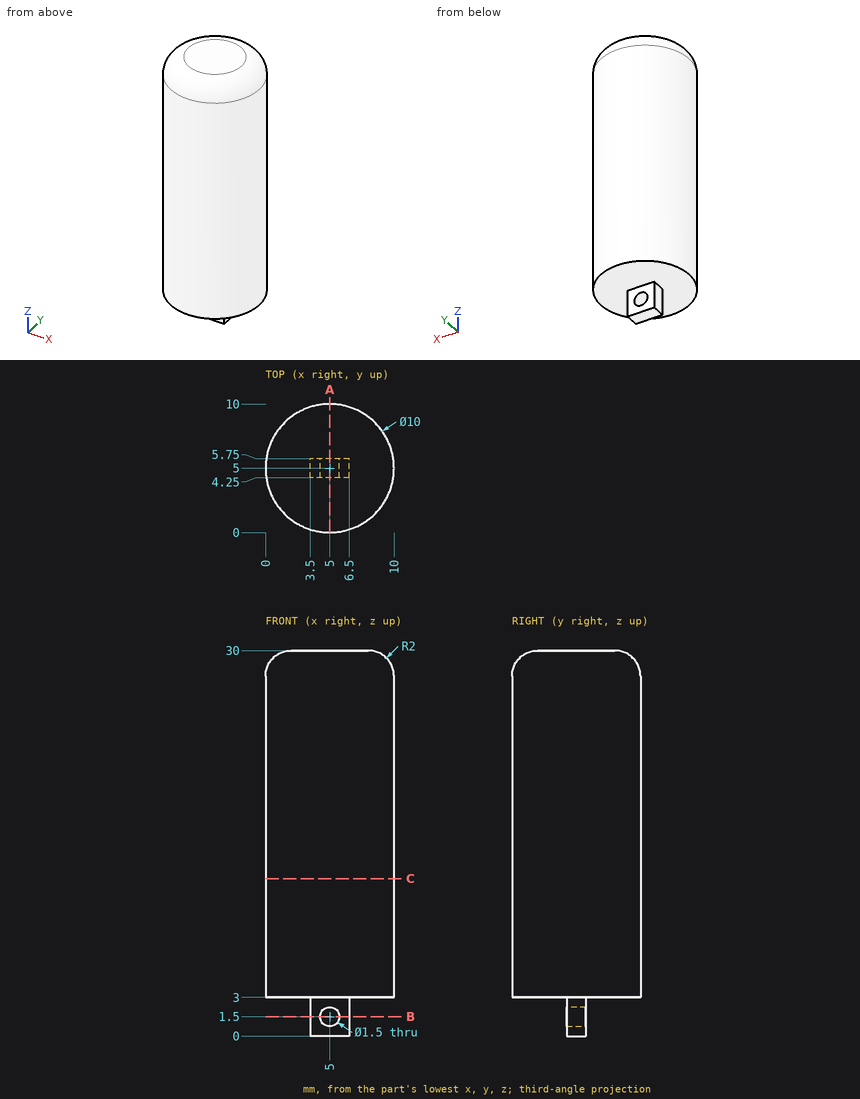
Print and shaded views of the part. All mm, measured from the part's lowest x, y and z. Round coordinates to 2 decimals unless told otherwise and drop trailing zeros. Write each loop counter-clockwise with the first axis right and the second up, starting at its lowest first coordinate (ties: lowest second). Pieces come first, ordered by that corner, then holes. Notation, with made-up numbers: (20.5, 86) - (77.5, 86) arc R34 cw to (77.5, 116) - close; hole circle Ø8 at (40, 5). An arc over 180 degrees is marked (long way). One line per question, with ' | ' between items.
1. Band-saw the part on B-B, the plane z = 1.5. Write the cut outline in (x, y).
Results are:
outline: (3.5, 4.25) - (4.25, 4.25) - (4.25, 5.75) - (3.5, 5.75) - close; (5.75, 4.25) - (6.5, 4.25) - (6.5, 5.75) - (5.75, 5.75) - close
2. Band-saw the part on C-C, the plane z = 12.25. Write the cut outline in (x, y), and give its area (3 significant figures).
Results are:
outline: circle Ø10 at (5, 5) | area: 78.5 mm^2
3. Drop flat-ended pins along their axis: pin 1 Ø1.5 at (x, z) = (5.5, 1) entering from +Y; pin 2 Ø2 at (x, y) = (5.5, 9) entering from -Z; pin 3 Ø4 at (y, z) = (9, 10) entering from -X. Give the stop position or say it passes through.
Results are:
pin 1: y = 5.75 | pin 2: z = 3 | pin 3: x = 0.42
4. Band-saw the part on A-A, the plane x = 5. Write the cut outline in (y, z).
Results are:
outline: (0, 3) - (4.25, 3) - (4.25, 2.25) - (5.75, 2.25) - (5.75, 3) - (10, 3) - (10, 28) arc R2 ccw to (8, 30) - (2, 30) arc R2 ccw to (0, 28) - close; (4.25, 0) - (5.75, 0) - (5.75, 0.75) - (4.25, 0.75) - close
5. Drill centre lines: line 1 along X through (y, z) = (4.8, 1.5); line 2 along Z through (x, y) = (7.25, 6); line 3 along X through (y, z) = (1, 5.75). Where is each one in solid material? Low to high. Write a range as from..to.
Results are:
line 1: 3.5..4.25, 5.75..6.5 | line 2: 3..30 | line 3: 2..8
